Geometry: final body of the model. Coordinates: model frame, mm. A direction names the side the tool comes from. Round coordinates to 2 decimals unless told otherwise and drop trailing zeros. Loops run counter-clockwise (first coordinate to the right, second up) from the corner with the lowest first, then second, coordinate; pieces in that order, holes last. Notation, with made-up numbers: (-33, 21.25) -> (-1, 21.25) arc R14 ccw to (-1, 40.25) -> close; hole circle Ø7 at (-22, -28.75). An arc over 180 degrees is marked (long way). Answer in a Markdown table with one row per item.
```python
from build123d import *

# Parameters (mm, degrees)
SKETCH_1_R           = 59.5
EXTRUDE_1_DEPTH      = 34.5
SKETCH_2_R           = 57.6
CUT_EXTRUDE_1_DEPTH  = 10.5
SKETCH_3_R           = 55.1
CUT_EXTRUDE_2_DEPTH  = 15.5
SKETCH_4_R           = 43
CUT_EXTRUDE_3_DEPTH  = 89.07099409
SKETCH_9_R           = 4
CUT_EXTRUDE_7_DEPTH  = 4
SKETCH_10_R          = 2.1
CUT_EXTRUDE_8_DEPTH  = 89.07099409
SKETCH_11_R          = 3.75
CUT_EXTRUDE_9_DEPTH  = 5
SKETCH_14_R          = 59.5
SKETCH_14_R_2        = 59.1
CUT_EXTRUDE_12_DEPTH = 91.94366388
CUT_EXTRUDE_13_DEPTH = 1


with BuildPart() as part:
    # 草图1 → 凸台-拉伸1 (new body)
    with BuildSketch(Plane(origin=(0, 0, 0), x_dir=(1, 0, 0), z_dir=(0, 1, 0))):
        with Locations(Location((0, 0, 0), (0, 0, 270))):
            Circle(SKETCH_1_R)
    extrude(amount=EXTRUDE_1_DEPTH)

    # 草图2 → 切除-拉伸1 (cut)
    with BuildSketch(Plane(origin=(0, 34.5, 0), x_dir=(1, 0, 0), z_dir=(0, 1, 0))):
        with Locations(Location((0, 0, 0), (0, 0, 270))):
            Circle(SKETCH_2_R)
    extrude(amount=-CUT_EXTRUDE_1_DEPTH, mode=Mode.SUBTRACT)

    # 草图3 → 切除-拉伸2 (cut)
    with BuildSketch(Plane(origin=(0, 24, 0), x_dir=(1, 0, 0), z_dir=(0, 1, 0))):
        with Locations(Location((0, 0, 0), (0, 0, 270))):
            Circle(SKETCH_3_R)
    extrude(amount=-CUT_EXTRUDE_2_DEPTH, mode=Mode.SUBTRACT)

    # 草图4 → 切除-拉伸3 (cut, through all)
    with BuildSketch(Plane(origin=(0, 8.5, 0), x_dir=(1, 0, 0), z_dir=(0, 1, 0))):
        with Locations(Location((0, 0, 0), (0, 0, 270))):
            Circle(SKETCH_4_R)
    extrude(amount=-CUT_EXTRUDE_3_DEPTH, mode=Mode.SUBTRACT)

    # 草图9 → 切除-拉伸7 (cut)
    with BuildSketch(Plane(origin=(0, 8.5, 0), x_dir=(1, 0, 0), z_dir=(0, 1, 0))):
        with Locations(Location((-44.167295593, 25.5, 0), (0, 0, 270))):
            Circle(SKETCH_9_R)
        with Locations(Location((-25.5, 44.167295593, 0), (0, 0, 270))):
            Circle(SKETCH_9_R)
        with Locations(Location((25.5, 44.167295593, 0), (0, 0, 270))):
            Circle(SKETCH_9_R)
        with Locations(Location((44.167295593, 25.5, 0), (0, 0, 270))):
            Circle(SKETCH_9_R)
        with Locations(Location((44.167295593, -25.5, 0), (0, 0, 270))):
            Circle(SKETCH_9_R)
        with Locations(Location((25.5, -44.167295593, 0), (0, 0, 270))):
            Circle(SKETCH_9_R)
        with Locations(Location((-25.5, -44.167295593, 0), (0, 0, 270))):
            Circle(SKETCH_9_R)
        with Locations(Location((-44.167295593, -25.5, 0), (0, 0, 270))):
            Circle(SKETCH_9_R)
    extrude(amount=-CUT_EXTRUDE_7_DEPTH, mode=Mode.SUBTRACT)

    # 草图10 → 切除-拉伸8 (cut, through all)
    with BuildSketch(Plane(origin=(0, 8.5, 0), x_dir=(1, 0, 0), z_dir=(0, 1, 0))):
        with Locations(Location((0, 51, 0), (0, 0, 270))):
            Circle(SKETCH_10_R)
        with Locations(Location((51, 0, 0), (0, 0, 270))):
            Circle(SKETCH_10_R)
        with Locations(Location((0, -51, 0), (0, 0, 270))):
            Circle(SKETCH_10_R)
        with Locations(Location((-51, 0, 0), (0, 0, 270))):
            Circle(SKETCH_10_R)
    extrude(amount=-CUT_EXTRUDE_8_DEPTH, mode=Mode.SUBTRACT)

    # 草图11 → 切除-拉伸9 (cut)
    with BuildSketch(Plane.XZ):
        with Locations(Location((0, 51, 0), (0, 0, 270))):
            Circle(SKETCH_11_R)
        with Locations(Location((51, 0, 0), (0, 0, 270))):
            Circle(SKETCH_11_R)
        with Locations(Location((0, -51, 0), (0, 0, 270))):
            Circle(SKETCH_11_R)
        with Locations(Location((-51, 0, 0), (0, 0, 270))):
            Circle(SKETCH_11_R)
    extrude(amount=-CUT_EXTRUDE_9_DEPTH, mode=Mode.SUBTRACT)

    # 草图14 → 切除-拉伸12 (cut, through all)
    with BuildSketch(Plane.XZ):
        Circle(SKETCH_14_R)
        with Locations(Location((0, 0, 0), (0, 0, 270))):
            Circle(SKETCH_14_R_2, mode=Mode.SUBTRACT)
    extrude(amount=-CUT_EXTRUDE_12_DEPTH, mode=Mode.SUBTRACT)

    # 草图15 → 切除-拉伸13 (cut)
    with BuildSketch(Plane.XZ):
        Polygon((0, -59.1), (0.5, -59.1), (0.5, -58.1), (-0.5, -58.1), (-0.5, -59.1), align=None)
        Polygon((0.5, 59.1), (0.5, 58.1), (-0.5, 58.1), (-0.5, 59.1), (0, 59.1), align=None)
    extrude(amount=-CUT_EXTRUDE_13_DEPTH, mode=Mode.SUBTRACT)


solid = part.part
```
Item 1: Cut plane A-A (z = 0). Count the separate pieces of the cut face and the enclosed holes in it, then the cut area to 3 significant figures.
Answer:
| item | result |
|---|---|
| separate pieces | 4 |
| enclosed holes | 0 |
| area | 325 mm² |
Item 2: Cut plane C-C (z = -51). Output: boundary loops of the cut face in (x, y), then the cut area to 3 significant figures.
Answer:
| item | result |
|---|---|
| outline | (-29.86, 0) -> (-3.75, 0) -> (-3.75, 5) -> (-2.1, 5) -> (-2.1, 8.5) -> (-20.86, 8.5) -> (-20.86, 24) -> (-26.77, 24) -> (-26.77, 34.5) -> (-29.86, 34.5) -> close; (2.1, 5) -> (3.75, 5) -> (3.75, 0) -> (29.86, 0) -> (29.86, 34.5) -> (26.77, 34.5) -> (26.77, 24) -> (20.86, 24) -> (20.86, 8.5) -> (2.1, 8.5) -> close |
| area | 800 mm² |
Item 3: Cut plane B-B (x = 36). Output: boundary loops of the cut face in (y, z), then the cut area to 3 significant figures.
Answer:
| item | result |
|---|---|
| outline | (0, -46.87) -> (34.5, -46.87) -> (34.5, -44.96) -> (24, -44.96) -> (24, -41.71) -> (8.5, -41.71) -> (8.5, -23.52) -> (0, -23.52) -> close; (0, 23.52) -> (8.5, 23.52) -> (8.5, 41.71) -> (24, 41.71) -> (24, 44.96) -> (34.5, 44.96) -> (34.5, 46.87) -> (0, 46.87) -> close |
| area | 597 mm² |
Item 4: Cut plane D-D (x = 51). Output: boundary loops of the cut face in (y, z), then the cut area to 3 significant figures.
Answer:
| item | result |
|---|---|
| outline | (0, -29.86) -> (34.5, -29.86) -> (34.5, -26.77) -> (24, -26.77) -> (24, -20.86) -> (8.5, -20.86) -> (8.5, -2.1) -> (5, -2.1) -> (5, -3.75) -> (0, -3.75) -> close; (0, 3.75) -> (5, 3.75) -> (5, 2.1) -> (8.5, 2.1) -> (8.5, 20.86) -> (24, 20.86) -> (24, 26.77) -> (34.5, 26.77) -> (34.5, 29.86) -> (0, 29.86) -> close |
| area | 800 mm² |
Item 5: Reachability of faces 3 (the face through (-22.127, 6.528, -42.017)), 4 (the face through (-0.8, 6.77, 52.94)), 5 (the face through (49, 5, -2)) from +Z, -Z, +X, -X, +Y, -Y: full face, straight path, thin tool, end or side. Return the list, or none.
Answer:
| item | result |
|---|---|
| face 3 | +Y |
| face 4 | +Y, -Y |
| face 5 | -Y |
Item 6: Pin query (flat end, axial travel): pin 1 Ø3.5 at (x, z) = (51, 0) entering from +Y; pin 2 Ø2.5 at (x, z) = (-23.5, 43.5) entering from +Y; pin 3 Ø0.5 at (x, z) = (0, 58.5) entering from -Y; pin 4 Ø7 at (x, z) = (0, 51) entering from -Y. Return the tip coordinate at first contact, or that it passes through.
Answer:
| item | result |
|---|---|
| pin 1 | passes through |
| pin 2 | stops at y = 4.5 |
| pin 3 | stops at y = 1 |
| pin 4 | stops at y = 5 |
Item 7: Draft query along X for faces 1 (the face through (47.34, 2.46, 0.81)), 2 (the face through (-30.4, 0, -30.9)). Return one class per face: pulls with the +X half, pulls with the -X half, needs draft (parallel to the pull), parting line crosses it, or undercut.
Answer:
| item | result |
|---|---|
| face 1 | undercut |
| face 2 | needs draft |
Item 8: Line query: probe 1 along X at (y, z) = (3.25, 0); probe 2 along X at (y, z) = (5, 25); probe 3 along X at (y, z) = (28.75, 0). Output: solid intervals per line, ascending. Write a range as [from, to].
Answer:
| item | result |
|---|---|
| probe 1 | x = [-59.1, -54.75], [-47.25, -43], [43, 47.25], [54.75, 59.1] |
| probe 2 | x = [-53.55, -48.14], [-40.2, -34.99], [34.99, 40.2], [48.14, 53.55] |
| probe 3 | x = [-59.1, -57.6], [57.6, 59.1] |
